```python
from build123d import *

# Parameters (mm, degrees)
BOSS_EXTRUDE1_DEPTH = 25.4
FILLET1_R           = 12.7
SKETCH2_R           = 6.35
CUT_EXTRUDE1_DEPTH  = 25.4
SKETCH3_R           = 3.175
CUT_EXTRUDE2_DEPTH  = 25.4


with BuildPart() as part:
    # Sketch1 → Boss-Extrude1 (new body)
    with BuildSketch(Plane(origin=(0, 0, 0), x_dir=(0, 0, -1), z_dir=(1, 0, 0))):
        with BuildLine():
            Line((-12.7, 0), (0, 0))
            Line((0, 0), (31.75, 0))
            Line((31.75, 0), (31.75, 6.35))
            Line((31.75, 6.35), (6.35, 6.35))
            ThreePointArc((6.35, 6.35), (1.859871939, 8.209871939), (0, 12.7))
            Line((0, 12.7), (0, 50.8))
            Line((0, 50.8), (-12.7, 50.8))
            Line((-12.7, 50.8), (-12.7, 0))
        make_face()
    extrude(amount=BOSS_EXTRUDE1_DEPTH)

    # Fillet1
    fillet1_edges = [part.edges().sort_by_distance(p)[0] for p in [
        (25.4, 50.8, 6.35),
        (0, 50.8, 6.35),
    ]]
    fillet(fillet1_edges, radius=FILLET1_R - 0.0001)  # a hair under: the kernel refuses the full size

    # Sketch2 → Cut-Extrude1 (cut)
    with BuildSketch(Plane.XY.offset(12.7)):
        with Locations((12.7, 38.1)):
            Circle(SKETCH2_R)
    extrude(amount=-CUT_EXTRUDE1_DEPTH, mode=Mode.SUBTRACT)

    # Sketch3 → Cut-Extrude2 (cut)
    with BuildSketch(Plane(origin=(0, 6.35, 0), x_dir=(1, 0, 0), z_dir=(0, 1, 0))):
        with Locations(Location((12.7, 25.4, 0), (0, 0, 270))):
            Circle(SKETCH3_R)
        with Locations(Location((12.7, 12.7, 0), (0, 0, 270))):
            Circle(SKETCH3_R)
    extrude(amount=-CUT_EXTRUDE2_DEPTH, mode=Mode.SUBTRACT)


solid = part.part
```
Geometry: final body of the model. Coordinates: model frame, mm. A direction names the side the tool comes from. Give positions to 0.01 mm unless a question says otherwise; leave off trailing zeros. Order: outer loops, then holes, each group sorted by start corner. A loop starts at its lowest first (then second) coordinate and runs counter-clockwise, first axis right, second up. Notation, with made-up numbers: (47.5, 51.25) -> (97.5, 51.25) arc R28 cw to (97.5, 85.25) -> close; hole circle Ø4 at (42.5, 89.5). An arc over 180 degrees is marked (long way). Write each question's results on one line, items separated by ' | '. Start each with the question number.
1) Line query: line 1 (Y direction, x = 12.7, z = 10); line 2 (X direction, y = 38, z = 8); line 3 (Y direction, x = 9.25, z = -9.5). Output: solid intervals per line, ascending. Write a range as from..to.
2) Section A-A (z = -25.4). Return loops of the section in (x, y) (3 decimals).
3) Set-up query: faces 5 (the flat face through (13, 6.35, -19)), 6 (the flat face through (13, 0, -9)). Return all of +Z, -Z, +X, -X, +Y, -Y with unobstructed straight access to the full face (end or side cutting, diameter ignored); none if empty.
4) First-contact query: pin 1 (3 mm diameter, centred on x = 10, z = -7, fed in from +Y); pin 2 (8 mm diameter, centred on x = 8.5, y = 38, fed in from +Z); pin 3 (10 mm diameter, centred on x = 12.7, z = -25.4, fed in from +Y); pin 4 (6 mm diameter, centred on x = 8.5, y = 19.5, fed in from -Z). Flat tips, straight axial feed; report the tip coordinate or a pass-through.
5) Draft query along Z for faces 1 (the cylindrical face through (9.9, 3.2, -11.2)), 2 (the flat face through (13, 27, 0)), 3 (the flat face through (25.4, 15, 1)), 4 (the cylindrical face through (11.48, 3.22, -22.47)). Return one class per face: pulls with the +Z half, pulls with the -Z half, needs draft (parallel to the pull), parting line crosses it, or undercut.
6) Section C-C (y = 33.5). Return loops of the section in (x, z), then the cut area to 3 significant figures.
7) Section D-D (x = 10.75). Return loops of the section in (y, z).
8) Section B-B (x = 16.75). Return loops of the section in (y, z).
Calculated:
1) line 1: 0..31.75, 44.45..50.8 | line 2: 0..6.35, 19.05..25.4 | line 3: 0..6.35
2) outline: (0, 0) -> (9.525, 0) -> (9.525, 6.35) -> (0, 6.35) -> close; (15.875, 0) -> (25.4, 0) -> (25.4, 6.35) -> (15.875, 6.35) -> close
3) face 5: -Z, +X, -X, +Y | face 6: +Z, -Z, +X, -X, -Y
4) pin 1: y = 6.41 | pin 2: z = 12.7 | pin 3: y = 6.35 | pin 4: z = 0
5) face 1: undercut | face 2: pulls with the -Z half | face 3: needs draft | face 4: undercut
6) outline: (0, 0) -> (8.32, 0) -> (8.32, 12.7) -> (0, 12.7) -> close; (17.08, 0) -> (25.4, 0) -> (25.4, 12.7) -> (17.08, 12.7) -> close | area: 211 mm2
7) outline: (0, -31.75) -> (6.35, -31.75) -> (6.35, -27.91) -> (0, -27.91) -> close; (0, -22.89) -> (6.35, -22.89) -> (6.35, -15.21) -> (0, -15.21) -> close; (0, -10.19) -> (6.35, -10.19) -> (6.35, -6.35) arc R6.35 cw to (12.7, 0) -> (32.06, 0) -> (32.06, 12.7) -> (0, 12.7) -> close; (44.14, 0) -> (50.65, 0) -> (50.65, 12.7) -> (44.14, 12.7) -> close
8) outline: (0, -31.75) -> (6.35, -31.75) -> (6.35, -6.35) arc R6.35 cw to (12.7, 0) -> (33.21, 0) -> (33.21, 12.7) -> (0, 12.7) -> close; (42.99, 0) -> (50.14, 0) -> (50.14, 12.7) -> (42.99, 12.7) -> close
